from build123d import *

# Parameters (mm, degrees)
SKETCH2_W           = 70
SKETCH2_H           = 54.7
SKETCH2_W_2         = 11
SKETCH2_H_2         = 11
SKETCH2_W_3         = 3.4
SKETCH2_W_4         = 9
SKETCH2_H_3         = 4.45
SKETCH2_R           = 2.6
BOSS_EXTRUDE1_DEPTH = 2


with BuildPart() as part:
    # Sketch2 → Boss-Extrude1 (new body)
    with BuildSketch(Plane(origin=(0, 0, 0), x_dir=(1, 0, 0), z_dir=(0, 1, 0))):
        with Locations((34, 26.35)):
            Rectangle(SKETCH2_W, SKETCH2_H)
        with Locations((22.25, 14.42)):
            Rectangle(SKETCH2_W_2, SKETCH2_H_2, mode=Mode.SUBTRACT)
        with Locations((32.95, 14.27)):
            Rectangle(SKETCH2_W_3, SKETCH2_H_2, mode=Mode.SUBTRACT)
        Polygon((18.25, 28.57), (22.75, 28.57), (27.25, 28.57), (27.25, 24.12), (22.75, 24.12), (18.25, 24.12), align=None, mode=Mode.SUBTRACT)
        with Locations((43.5, 14.42)):
            Rectangle(SKETCH2_W_2, SKETCH2_H_2, mode=Mode.SUBTRACT)
        with Locations((44, 26.345)):
            Rectangle(SKETCH2_W_4, SKETCH2_H_3, mode=Mode.SUBTRACT)
        with Locations((54.2, 14.27)):
            Rectangle(SKETCH2_W_3, SKETCH2_H_2, mode=Mode.SUBTRACT)
        Polygon((67.5, 4), (61.5, 4), (61.5, 37.45), (58, 37.45), (58, 48.45), (64, 48.45), (64, 38), (67.5, 38), align=None, mode=Mode.SUBTRACT)
        with Locations((22.25, 38.57)):
            Rectangle(SKETCH2_W_2, SKETCH2_H_2, mode=Mode.SUBTRACT)
        with Locations((32.95, 38.42)):
            Rectangle(SKETCH2_W_3, SKETCH2_H_2, mode=Mode.SUBTRACT)
        with Locations((5, 48.7)):
            Circle(SKETCH2_R, mode=Mode.SUBTRACT)
        with Locations((43.5, 38.57)):
            Rectangle(SKETCH2_W_2, SKETCH2_H_2, mode=Mode.SUBTRACT)
        with Locations((54.2, 38.42)):
            Rectangle(SKETCH2_W_3, SKETCH2_H_2, mode=Mode.SUBTRACT)
    extrude(amount=BOSS_EXTRUDE1_DEPTH)


solid = part.part
Design review of the part built by this model. Coordinates are the model's own, in mm. Give positions to 0.01 mm unless a question says otherwise; leave off trailing zeros. Loops run counter-clockwise (first coordinate to the right, second up) from the corner with the lowest first, then second, coordinate; pieces in that order, holes last. Notation, with made-up numbers: M 84,-7 L 96,-7 A24 cw 96,16 Z; hole C 23.25,-3.75 d5. An arc over 180 degrees is marked long. One line per question, with ' | ' between items. Start each with the question number.
1. Add section A-A (x = 5). Write out the cut boundary in (y, z), plus the area to 3 significant figures.
2. Add section D-D (x = 19.5). Write out the cut boundary in (y, z).
3. Add section B-B (z = -27). Write out the cut boundary in (x, y).
4. The part is to be moulded in two halves that separate along X. For faces 1 (the face through (16.75, 1, -38)), 2 (the face through (34, 0, -27)), say which applies: released by +X, released by -X, zero draft, split by the parting line, or undercut.
5. Add section C-C (z = -11). Write out the cut boundary in (x, y), plus the area to 3 significant figures.
6. To check wall thickness, follow L1, parallel to X at y = 1.8, z = -25.5; L2, parallel to Z at x = 38.5, y = 1.15; L3, parallel to Z at x = 27, y = 1.45. State the ranges of each line that lie inside material, in increasing order.
Worked out:
1) outline: M 0,-53.7 L 2,-53.7 L 2,-51.3 L 0,-51.3 Z; M 0,-46.1 L 2,-46.1 L 2,1 L 0,1 Z | area: 99.0 mm²
2) outline: M 0,-53.7 L 2,-53.7 L 2,-44.07 L 0,-44.07 Z; M 0,-33.07 L 2,-33.07 L 2,-28.57 L 0,-28.57 Z; M 0,-24.12 L 2,-24.12 L 2,-19.92 L 0,-19.92 Z; M 0,-8.92 L 2,-8.92 L 2,1 L 0,1 Z
3) outline: M -1,0 L 18.25,0 L 18.25,2 L -1,2 Z; M 27.25,0 L 39.5,0 L 39.5,2 L 27.25,2 Z; M 48.5,0 L 61.5,0 L 61.5,2 L 48.5,2 Z; M 67.5,0 L 69,0 L 69,2 L 67.5,2 Z
4) face 1: undercut | face 2: zero draft
5) outline: M -1,0 L 16.75,0 L 16.75,2 L -1,2 Z; M 27.75,0 L 31.25,0 L 31.25,2 L 27.75,2 Z; M 34.65,0 L 38,0 L 38,2 L 34.65,2 Z; M 49,0 L 52.5,0 L 52.5,2 L 49,2 Z; M 55.9,0 L 61.5,0 L 61.5,2 L 55.9,2 Z; M 67.5,0 L 69,0 L 69,2 L 67.5,2 Z | area: 70.4 mm²
6) L1: x = -1 to 18.25, 27.25 to 39.5, 48.5 to 61.5, 67.5 to 69 | L2: z = -53.7 to -44.07, -33.07 to -19.92, -8.92 to 1 | L3: z = -53.7 to -44.07, -33.07 to -28.57, -24.12 to -19.92, -8.92 to 1
